Here's how the part is built. I have some questions about the finished solid (model axes, mm). Round coordinates to 2 decimals unless told otherwise and drop trailing zeros. Write each loop counter-clockwise with the first axis right and the second up, starting at its lowest first coordinate (ties: lowest second). Pieces come first, ordered by that corner, then holes. Notation, with made-up numbers: (0, 30.25) -> (19, 30.25) arc R36 cw to (19, 64.25) -> close; hole circle Ø9 at (30.5, -20.5). An arc over 180 degrees is marked (long way). Answer in a Markdown table with one row per item.
from build123d import *

# Parameters (mm, degrees)
F0_R     = 76.2
F1_DEPTH = 50.8
F3_R     = 19.05
F4_DEPTH = 50.801
F5_R     = 6.35
F6_DEPTH = 50.8010001


with BuildPart() as f1:
    # F0 (on Front) → F1 (new body)
    with BuildSketch(Plane.XZ):
        Circle(F0_R)
    extrude(amount=F1_DEPTH)

    # F3
    f3_edges = [f1.edges().sort_by_distance(p)[0] for p in [
        (76.2, -25.4, 0),
        (-76.2, 0, 0),
        (-76.2, -50.8, 0),
    ]]
    fillet(f3_edges, radius=F3_R)

    # F2 (on face) → F4 (cut, through all)
    with BuildSketch(Plane.XZ.offset(50.8)):
        with BuildLine():
            ThreePointArc((-29.6171166047, 29.6171166047), (-12.2470246704, 51.2799506522), (0, 76.2))
            Line((0, 76.2), (-38.1, 38.1))
            Line((-38.1, 38.1), (-29.6171166047, 29.6171166047))
        make_face()
        with BuildLine():
            Line((-29.6171166047, 29.6171166047), (-38.1, 38.1))
            Line((-38.1, 38.1), (-76.2, 0))
            ThreePointArc((-76.2, 0), (-51.2799506522, 12.2470246704), (-29.6171166047, 29.6171166047))
        make_face()
        with BuildLine():
            Line((0, -76.2), (38.1, -38.1))
            Line((38.1, -38.1), (29.6171166047, -29.6171166047))
            ThreePointArc((29.6171166047, -29.6171166047), (12.2470246704, -51.2799506522), (0, -76.2))
        make_face()
        with BuildLine():
            Line((38.1, -38.1), (76.2, 0))
            ThreePointArc((76.2, 0), (51.2799506522, -12.2470246704), (29.6171166047, -29.6171166047))
            Line((29.6171166047, -29.6171166047), (38.1, -38.1))
        make_face()
        with BuildLine():
            ThreePointArc((29.6171166047, 29.6171166047), (51.2799506522, 12.2470246704), (76.2, 0))
            Line((76.2, 0), (38.1, 38.1))
            Line((38.1, 38.1), (29.6171166047, 29.6171166047))
        make_face()
        with BuildLine():
            Line((38.1, 38.1), (0, 76.2))
            ThreePointArc((0, 76.2), (12.2470246704, 51.2799506522), (29.6171166047, 29.6171166047))
            Line((29.6171166047, 29.6171166047), (38.1, 38.1))
        make_face()
        with BuildLine():
            ThreePointArc((-29.6171166047, -29.6171166047), (-51.2799506522, -12.2470246704), (-76.2, 0))
            Line((-76.2, 0), (-38.1, -38.1))
            Line((-38.1, -38.1), (-29.6171166047, -29.6171166047))
        make_face()
        with BuildLine():
            Line((-38.1, -38.1), (0, -76.2))
            ThreePointArc((0, -76.2), (-12.2470246704, -51.2799506522), (-29.6171166047, -29.6171166047))
            Line((-29.6171166047, -29.6171166047), (-38.1, -38.1))
        make_face()
        with BuildLine():
            Line((53.8815367264, 53.8815367264), (76.2, 76.2))
            Line((76.2, 76.2), (0, 76.2))
            ThreePointArc((0, 76.2), (29.1604775462, 70.3996203774), (53.8815367264, 53.8815367264))
        make_face()
        with BuildLine():
            ThreePointArc((-53.8815367264, 53.8815367264), (-29.1604775462, 70.3996203774), (0, 76.2))
            Line((0, 76.2), (-76.2, 76.2))
            Line((-76.2, 76.2), (-53.8815367264, 53.8815367264))
        make_face()
        with BuildLine():
            Line((0, -76.2), (76.2, -76.2))
            Line((76.2, -76.2), (53.8815367264, -53.8815367264))
            ThreePointArc((53.8815367264, -53.8815367264), (29.1604775462, -70.3996203774), (0, -76.2))
        make_face()
        with BuildLine():
            Line((-76.2, -76.2), (0, -76.2))
            ThreePointArc((0, -76.2), (-29.1604775462, -70.3996203774), (-53.8815367264, -53.8815367264))
            Line((-53.8815367264, -53.8815367264), (-76.2, -76.2))
        make_face()
        with BuildLine():
            Line((76.2, 0), (76.2, 76.2))
            Line((76.2, 76.2), (53.8815367264, 53.8815367264))
            ThreePointArc((53.8815367264, 53.8815367264), (70.3996203774, 29.1604775462), (76.2, 0))
        make_face()
        with BuildLine():
            Line((76.2, -76.2), (76.2, 0))
            ThreePointArc((76.2, 0), (70.3996203774, -29.1604775462), (53.8815367264, -53.8815367264))
            Line((53.8815367264, -53.8815367264), (76.2, -76.2))
        make_face()
        with BuildLine():
            Line((-53.8815367264, 53.8815367264), (-76.2, 76.2))
            Line((-76.2, 76.2), (-76.2, 0))
            ThreePointArc((-76.2, 0), (-70.3996203774, 29.1604775462), (-53.8815367264, 53.8815367264))
        make_face()
        with BuildLine():
            ThreePointArc((-53.8815367264, -53.8815367264), (-70.3996203774, -29.1604775462), (-76.2, 0))
            Line((-76.2, 0), (-76.2, -76.2))
            Line((-76.2, -76.2), (-53.8815367264, -53.8815367264))
        make_face()
        with BuildLine():
            Line((-38.1, 38.1), (0, 76.2))
            ThreePointArc((0, 76.2), (-29.1604775462, 70.3996203774), (-53.8815367264, 53.8815367264))
            Line((-53.8815367264, 53.8815367264), (-38.1, 38.1))
        make_face()
        with BuildLine():
            Line((-76.2, 0), (-38.1, 38.1))
            Line((-38.1, 38.1), (-53.8815367264, 53.8815367264))
            ThreePointArc((-53.8815367264, 53.8815367264), (-70.3996203774, 29.1604775462), (-76.2, 0))
        make_face()
        with BuildLine():
            Line((53.8815367264, -53.8815367264), (38.1, -38.1))
            Line((38.1, -38.1), (0, -76.2))
            ThreePointArc((0, -76.2), (29.1604775462, -70.3996203774), (53.8815367264, -53.8815367264))
        make_face()
        with BuildLine():
            ThreePointArc((53.8815367264, -53.8815367264), (70.3996203774, -29.1604775462), (76.2, 0))
            Line((76.2, 0), (38.1, -38.1))
            Line((38.1, -38.1), (53.8815367264, -53.8815367264))
        make_face()
        with BuildLine():
            Line((38.1, 38.1), (76.2, 0))
            ThreePointArc((76.2, 0), (70.3996203774, 29.1604775462), (53.8815367264, 53.8815367264))
            Line((53.8815367264, 53.8815367264), (38.1, 38.1))
        make_face()
        with BuildLine():
            ThreePointArc((53.8815367264, 53.8815367264), (29.1604775462, 70.3996203774), (0, 76.2))
            Line((0, 76.2), (38.1, 38.1))
            Line((38.1, 38.1), (53.8815367264, 53.8815367264))
        make_face()
        with BuildLine():
            Line((-38.1, -38.1), (-76.2, 0))
            ThreePointArc((-76.2, 0), (-70.3996203774, -29.1604775462), (-53.8815367264, -53.8815367264))
            Line((-53.8815367264, -53.8815367264), (-38.1, -38.1))
        make_face()
        with BuildLine():
            ThreePointArc((-53.8815367264, -53.8815367264), (-29.1604775462, -70.3996203774), (0, -76.2))
            Line((0, -76.2), (-38.1, -38.1))
            Line((-38.1, -38.1), (-53.8815367264, -53.8815367264))
        make_face()
    extrude(amount=-F4_DEPTH, mode=Mode.SUBTRACT)

    # F5 (on face) → F6 (cut, through all)
    with BuildSketch(Plane.XZ.offset(50.8)):
        Circle(F5_R)
    extrude(amount=-F6_DEPTH, mode=Mode.SUBTRACT)


solid = f1.part
1) I want a section at D-D, the plane x = 46. List the corners of the cut face in (y, z) for me.
Response:
| item | result |
|---|---|
| outline | (-50.8, -15.79) -> (0, -15.79) -> (0, 15.79) -> (-50.8, 15.79) -> close |
2) We'd pull the mould along X, two halves only. Please class faces 1 (the face through (-1.38, -25.76, -6.2)), 2 (the face through (12, 0, 1)): +X half, -X half, draft (parallel to the pull), parting line (faces both ways), or undercut.
Response:
| item | result |
|---|---|
| face 1 | undercut |
| face 2 | draft |
3) I want a section at C-C, the plane y = -47. List the corners of the cut face in (x, z) for me, and give its area (3 significant figures).
Response:
| item | result |
|---|---|
| outline | (-68.5, -3.08) arc R127 cw to (-3.08, -68.5) arc R68.57 ccw to (3.08, -68.5) arc R127 cw to (68.5, -3.08) arc R68.57 ccw to (68.5, 3.08) arc R127 cw to (3.08, 68.5) arc R68.57 ccw to (-3.08, 68.5) arc R127 cw to (-68.5, 3.08) arc R68.57 ccw to start; hole circle Ø12.7 at (0, 0) |
| area | 7,910 mm^2 |
4) I want a section at B-B, the plane z = 13. List the corners of the cut face in (x, y) for me, and give its area (3 significant figures).
Response:
| item | result |
|---|---|
| outline | (-50.11, -50.8) -> (50.11, -50.8) -> (50.11, 0) -> (-50.11, 0) -> close |
| area | 5,090 mm^2 |
5) I need wall thicknesses on line 1 (Z direction, x = 0, y = -36); line 2 (Z direction, x = 2.5, y = -13); line 3 (X direction, y = -33, z = -24). Which ranges of each line are inside material? Lowest first, please. Write a range as [from, to].
Response:
| item | result |
|---|---|
| line 1 | z = [-75.72, -6.35], [6.35, 75.72] |
| line 2 | z = [-69.83, -5.84], [5.84, 69.83] |
| line 3 | x = [-35.61, 35.61] |
6) For pin 1 (2 mm diameter, centred on x = 15, y = -42.5, fed in from -Z); pin 2 (10 mm diameter, centred on y = -11.5, z = 60, fed in from -X); pin 3 (10 mm diameter, centred on x = -5, y = -10.5, fed in from +Z), each with a flat end and sliding along its axis, tell me the tip position at first contact or that it passes through.
Response:
| item | result |
|---|---|
| pin 1 | stops at z = -48.6 |
| pin 2 | stops at x = -9.97 |
| pin 3 | stops at z = 75.04 |
7) I want a section at A-A, the plane y = -25. List the corners of the cut face in (x, z) for me, and give its area (3 significant figures).
Response:
| item | result |
|---|---|
| outline | (-76.2, 0) arc R127 cw to (0, -76.2) arc R127 cw to (76.2, 0) arc R127 cw to (0, 76.2) arc R127 cw to start; hole circle Ø12.7 at (0, 0) |
| area | 8,000 mm^2 |
